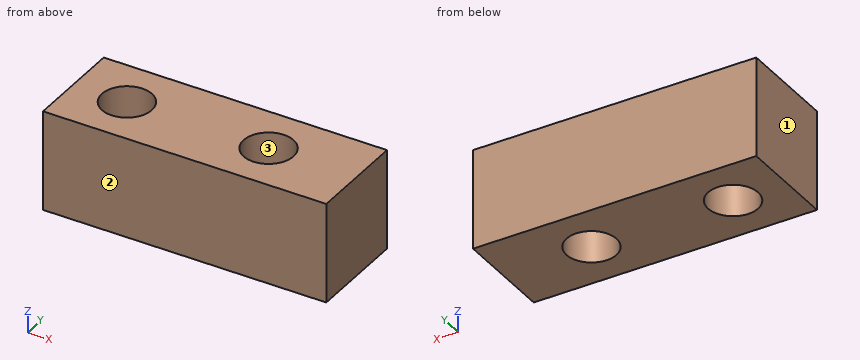
Autodesk Inventor part; units mm, degrees
ref_plane "YZ Plane" through (0, 0, 0) normal (1, 0, 0) x (0, 1, 0)
ref_plane "XZ Plane" through (0, 0, 0) normal (0, 1, 0) x (-1, 0, 0)
ref_plane "XY Plane" through (0, 0, 0) normal (0, 0, 1) x (1, 0, 0)
sketch "Sketch1" plane through (0, 0, 0) normal (0, 0, 1) x (1, 0, 0)
  circle A0 centre (-13.7859, 3) radius 1.5
  circle A1 centre (-5.2859, 3) radius 1.5
  line L0 (0, 0) -> (-17, 0)
  line L1 (0, 6) -> (0, 0)
  line L2 (-17, 6) -> (0, 6)
  line L3 (-17, 0) -> (-17, 6)
extrude "Extrusion1" add sketch "Sketch1" along normal blind 6
properties part number "XcrRightXEndstopTrigger"
The model under review builds one solid part; all positions refer to its coordinate system, in mm. Face numbers are marked on the shaded views. Give positions to 0.01 mm unless a question says otherwise; leave off trailing zeros. Order: outer loops, then holes, each group sorted by start corner. A loop starts at its lowest first (then second) coordinate and runs counter-clockwise, first axis right, second up. Notation, with made-up numbers: M -18.75,8.25 L -9.75,8.25 A18 ccw -9.75,29.25 Z; hole C -10,66.25 d11. An arc over 180 degrees is marked long. Use one line per item in the form item = value. Start each with the question number.
Item 1: The part is to be moulded in two halves that separate along X. For the marked faces 1, 2 and 3, say which applies: pulls with the +X half, pulls with the -X half, needs draft (parallel to the pull), parting line crosses it, or undercut.
Item 2: We need section D-D on y = 2.2. Give the boundary of the cut face in (x, z).
Item 3: To check wall thickness, follow line 1 along X through (y, z) = (3.4, 0.6); line 2 along Y through (x, z) = (-4.5, 2.9); line 3 along X through (y, z) = (2.4, 4.75). State the ranges of each line that lie inside material, in increasing order. Write a range as from..to.
Item 4: We need section B-B on x = -14.75. Give the boundary of the cut face in (y, z).
Item 5: We need section C-C on z = 1.15. Give the boundary of the cut face in (x, y), plus the area to 3 significant figures.
Item 6: Insertion check: pin 1 Ø2.5 at (x, y) = (-5.29, 3) entering from -Z. The pin has a flat end and moves straight along its axis. Give the tip position at first contact, or say it passes through.
Item 7: We need section A-A on y = 3. Give the boundary of the cut face in (x, z).
Completed:
q1.face_1 = pulls with the -X half
q1.face_2 = needs draft
q1.face_3 = undercut
q2.outline = M -17,0 L -15.05,0 L -15.05,6 L -17,6 Z; M -12.52,0 L -6.55,0 L -6.55,6 L -12.52,6 Z; M -4.02,0 L 0,0 L 0,6 L -4.02,6 Z
q3.line_1 = -17..-15.23, -12.34..-6.73, -3.84..0
q3.line_2 = 0..1.72, 4.28..6
q3.line_3 = -17..-15.16, -12.41..-6.66, -3.91..0
q4.outline = M 0,0 L 1.85,0 L 1.85,6 L 0,6 Z; M 4.15,0 L 6,0 L 6,6 L 4.15,6 Z
q5.outline = M -17,0 L 0,0 L 0,6 L -17,6 Z; hole C -13.79,3 d3; hole C -5.29,3 d3
q5.area = 87.9 mm²
q6.pin_1 = through
q7.outline = M -17,0 L -15.29,0 L -15.29,6 L -17,6 Z; M -12.29,0 L -6.79,0 L -6.79,6 L -12.29,6 Z; M -3.79,0 L 0,0 L 0,6 L -3.79,6 Z
